```python
from build123d import *

# Parameters (mm, degrees)
BOSS_EXTRUDE1_DEPTH = 1524


with BuildPart() as part:
    # Sketch1 → Boss-Extrude1 (new body)
    with BuildSketch(Plane.XY):
        with BuildLine():
            Line((-36.22675, 20.6375), (-3.46075, 20.6375))
            ThreePointArc((-3.46075, 20.6375), (-1.013630207, 19.623869793), (0, 17.17675))
            Line((0, 17.17675), (0, -17.17675))
            ThreePointArc((0, -17.17675), (-1.013630207, -19.623869793), (-3.46075, -20.6375))
            Line((-3.46075, -20.6375), (-36.22675, -20.6375))
            ThreePointArc((-36.22675, -20.6375), (-39.796401808, -19.158901808), (-41.275, -15.58925))
            Line((-41.275, -15.58925), (-41.275, -14.57325))
            ThreePointArc((-41.275, -14.57325), (-40.261369793, -12.126130207), (-37.81425, -11.1125))
            Line((-37.81425, -11.1125), (-35.5346, -11.1125))
            ThreePointArc((-35.5346, -11.1125), (-34.1376, -12.5095), (-35.5346, -13.9065))
            Line((-35.5346, -13.9065), (-37.81425, -13.9065))
            ThreePointArc((-37.81425, -13.9065), (-38.285713446, -14.101786554), (-38.481, -14.57325))
            Line((-38.481, -14.57325), (-38.481, -15.58925))
            ThreePointArc((-38.481, -15.58925), (-37.820745461, -17.183245461), (-36.22675, -17.8435))
            Line((-36.22675, -17.8435), (-3.46075, -17.8435))
            ThreePointArc((-3.46075, -17.8435), (-2.989286554, -17.648213446), (-2.794, -17.17675))
            Line((-2.794, -17.17675), (-2.794, 17.17675))
            ThreePointArc((-2.794, 17.17675), (-2.989286554, 17.648213446), (-3.46075, 17.8435))
            Line((-3.46075, 17.8435), (-36.22675, 17.8435))
            ThreePointArc((-36.22675, 17.8435), (-37.820745461, 17.183245461), (-38.481, 15.58925))
            Line((-38.481, 15.58925), (-38.481, 14.57325))
            ThreePointArc((-38.481, 14.57325), (-38.285713446, 14.101786554), (-37.81425, 13.9065))
            Line((-37.81425, 13.9065), (-35.5346, 13.9065))
            ThreePointArc((-35.5346, 13.9065), (-34.1376, 12.5095), (-35.5346, 11.1125))
            Line((-35.5346, 11.1125), (-37.81425, 11.1125))
            ThreePointArc((-37.81425, 11.1125), (-40.261369793, 12.126130207), (-41.275, 14.57325))
            Line((-41.275, 14.57325), (-41.275, 15.58925))
            ThreePointArc((-41.275, 15.58925), (-39.796401808, 19.158901808), (-36.22675, 20.6375))
        make_face()
    extrude(amount=-BOSS_EXTRUDE1_DEPTH)


with BuildPart() as body_2:
    # Mirror1: mirrored copy
    add(part.part.mirror(Plane(origin=(0, 17.17675, -1524), x_dir=(0, 0, 1), z_dir=(1, 0, 0))))

    # Combine1: union part
    add(part.part)


solid = body_2.part
```
Input: part model. Units: mm. Frame: model coordinates. A direction names the side the tool comes from. Coordinates: 2 decimals unless noted, no trailing zeros. Loops run counter-clockwise (first coordinate to the right, second up) from the corner with the lowest first, then second, coordinate; pieces in that order, holes last. Notation, with made-up numbers: M 89,11 L 120,11 A14 cw 120,19 Z; hole C -39,-19.5 d7. An arc over 180 degrees is marked long. Answer in a Markdown table with one row per item.
1. Draft query along X for faces 1 (the flat face through (2.794, 0, -751)), 2 (the flat face through (20, -20.638, -751)). Return one class per face: pulls with the +X half, pulls with the -X half, needs draft (parallel to the pull), parting line crosses it, or undercut.
Response:
| item | result |
|---|---|
| face 1 | undercut |
| face 2 | needs draft |
2. Reachability of faces 3 (the flat face through (20, 20.638, -751)), 4 (the flat face through (20, -17.844, -751)) from +Z, -Z, +X, -X, +Y, -Y: full face, straight path, thin tool, end or side. Return the list, or none.
Response:
| item | result |
|---|---|
| face 3 | +Z, -Z, +X, -X, +Y |
| face 4 | +Z, -Z |
3. Material intervals for line 1 (Y direction, x = 35.5, z = -1401.5); line 2 (Y direction, x = 37.5, z = -779); line 3 (Y direction, x = -29.5, z = -776), sorted ascending.
Response:
| item | result |
|---|---|
| line 1 | y = -20.64 to -17.84, -13.91 to -11.11, 11.11 to 13.91, 17.84 to 20.64 |
| line 2 | y = -20.47 to -17.45, -13.91 to -11.11, 11.11 to 13.91, 17.45 to 20.47 |
| line 3 | y = -20.64 to -17.84, 17.84 to 20.64 |
4. Section A-A, the plane y = 3. Output: boundary loops of the cut face in (x, z), then the cut area to 3 significant figures.
Response:
| item | result |
|---|---|
| outline | M -2.79,-1524 L 2.79,-1524 L 2.79,0 L -2.79,0 Z |
| area | 8,520 mm2 |
5. First-contact query: pin 1 (2 mm diameter, centred on y = -3.5, z = -740.5, fed in from +X); pin 2 (1.1 mm diameter, centred on x = -37, z = -1109.5, fed in from -Y); pin 3 (0.7 mm diameter, centred on x = -37, z = -573, fed in from +Y); pin 4 (6 mm diameter, centred on x = -4.5, y = 4, fed in from -Z). Flat tips, straight axial feed; report the tip coordinate or a pass-through.
Response:
| item | result |
|---|---|
| pin 1 | stops at x = 2.79 |
| pin 2 | stops at y = -20.63 |
| pin 3 | stops at y = 20.62 |
| pin 4 | stops at z = -1524 |
